Autodesk Inventor part; units mm, degrees
ref_plane "YZ Plane" through (0, 0, 0) normal (1, 0, 0) x (0, 1, 0)
ref_plane "XZ Plane" through (0, 0, 0) normal (0, 1, 0) x (-1, 0, 0)
ref_plane "XY Plane" through (0, 0, 0) normal (0, 0, 1) x (1, 0, 0)
sketch "Sketch1" plane through (0, 0, 0) normal (0, 1, 0) x (-1, 0, 0)
  line L0 (0, 0) -> (-38.1, 0)
  line L1 (-38.1, 0) -> (-38.1, -38.1)
  line L2 (-38.1, -38.1) -> (0, -38.1)
  line L3 (0, -38.1) -> (0, 0)
  dimension "d0" = 38.1
  dimension "d1" = 38.1
extrude "Extrusion1" add sketch "Sketch1" along normal blind 7.62
sketch "Sketch2" plane through (0, 7.62, 0) normal (0, 1, 0) x (1, 0, 0)
  line L0 (4.5036, 33.196) -> (33.3072, 33.196)
  line L1 (33.3072, 33.196) -> (33.3072, 4.3924)
  line L2 (33.3072, 4.3924) -> (4.5036, 4.3924)
  line L3 (4.5036, 4.3924) -> (4.5036, 33.196)
  line L4 (33.3072, 33.196) -> (4.5036, 4.3924)
  line L5 (4.5036, 33.196) -> (33.3072, 4.3924)
  line L6 (18.9054, 18.7942) -> (27.1672, 27.056)
  line L7 (18.9054, 18.7942) -> (10.6436, 27.056)
  line L8 (18.9054, 18.7942) -> (10.6436, 10.5324)
  line L9 (18.9054, 18.7942) -> (27.1672, 10.5324)
  line L10 (18.9054, 18.7942) -> (31.2263, 31.1151)
  line L11 (18.9054, 18.7942) -> (6.5845, 31.1151)
  line L12 (18.9054, 18.7942) -> (6.5845, 6.4733)
  line L13 (18.9054, 18.7942) -> (31.2263, 6.4733)
  circle A0 centre (27.1672, 27.056) radius 0.508
  circle A1 centre (31.2263, 31.1151) radius 0.508
  circle A2 centre (6.5845, 31.1151) radius 0.508
  circle A3 centre (10.6436, 27.056) radius 0.508
  circle A4 centre (10.6436, 10.5324) radius 0.508
  circle A5 centre (6.5845, 6.4733) radius 0.508
  line L14 (18.9054, 18.7942) -> (27.1672, 10.5324)
  circle A6 centre (27.1672, 10.5324) radius 0.508
  circle A7 centre (31.2263, 6.4733) radius 0.508
  circle A8 centre (18.9054, 18.7942) radius 4.1783
  point P0 (0, 0)
  point P1 (27.2554, -7.62)
  dimension "d4" = 28.8036
  dimension "d5" = 28.8036
  dimension "d6" = 11.684
  dimension "d7" = 11.684
  dimension "d8" = 11.684
  dimension "d9" = 17.4244
  dimension "d10" = 17.4244
  dimension "d11" = 17.4244
  dimension "d12" = 17.4244
  dimension "d13" = 1.016
  dimension "d14" = 1.016
  dimension "d15" = 1.016
  dimension "d16" = 1.016
  dimension "d17" = 1.016
  dimension "d18" = 1.016
  dimension "d19" = 11.684
  dimension "d20" = 1.016
  dimension "d21" = 1.016
  dimension "d22" = 8.3566
extrude "Extrusion2" cut sketch "Sketch2" against normal blind 25.4 contours A2 L5 | L5 A2 | A1 L4 | L4 A1 | A5 L4 | L4 A5 | A7 L5 | L5 A7 | A3 L5 | L5 A3 | A0 L4 | L4 A0 | A4 L4 | L4 A4 | A6 L5 | L5 A6 | A8 L4 L5 | L5 L4 A8 | A8 L5 L4 | L4 L5 A8
fillet "Fillet1" radius 6.35 4 edges at (38.1, 3.81, 0) (0, 3.81, 0) (0, 3.81, -38.1) (38.1, 3.81, -38.1)
Verification items for the finished model (mm, model axes). Round coordinates to 2 decimals unless told otherwise and drop trailing zeros. Write each loop counter-clockwise with the first axis right and the second up, starting at its lowest first coordinate (ties: lowest second). Pieces come first, ordered by that corner, then holes.
(1) Section check D-D (z = -2.5). Enter the section's corners in (x, y).
Returned:
outline: (1.3, 0) - (36.8, 0) - (36.8, 7.62) - (1.3, 7.62) - close
(2) Section check A-A (z = -21.5). Enter the section's corners in (x, y).
Returned:
outline: (0, 0) - (15.72, 0) - (15.72, 7.62) - (0, 7.62) - close; (22.09, 0) - (38.1, 0) - (38.1, 7.62) - (22.09, 7.62) - close
(3) Mould release check, pull along Z, two halves, no side actions. Record for faces 1 (the flat face through (19, 4, -38.1)), 2 (the cylindrical face through (27.636, 3.863, -10.338)), 3 (the flat face through (24, 7.62, -19)): pulls with the +Z half, pulls with the -Z half, needs draft (parallel to the pull), parting line crosses it, or undercut.
Returned:
face 1: pulls with the -Z half
face 2: undercut
face 3: needs draft
(4) Material ranges on line 1 (X direction, y = 6, z = -10.5); line 2 (Z direction, x = 10.5, y = 3.75); line 3 (Z direction, x = 16, y = 1.25), recorded low to high.
Returned:
line 1: x = 0 to 10.14, 11.15 to 26.66, 27.67 to 38.1
line 2: z = -38.1 to -27.54, -26.57 to -11.02, -10.05 to 0
line 3: z = -38.1 to -21.8, -15.79 to 0
(5) Section check C-C (x = 15.5). Enter the section's corners in (y, z).
Returned:
outline: (0, -38.1) - (7.62, -38.1) - (7.62, -21.22) - (0, -21.22) - close; (0, -16.37) - (7.62, -16.37) - (7.62, 0) - (0, 0) - close
(6) Section check B-B (y = 3.5). Give the number of separate pieces and of enclosed holes in the cut face, plus the area to 3 significant figures.
Returned:
separate pieces: 1
enclosed holes: 9
area: 1,360 mm2
